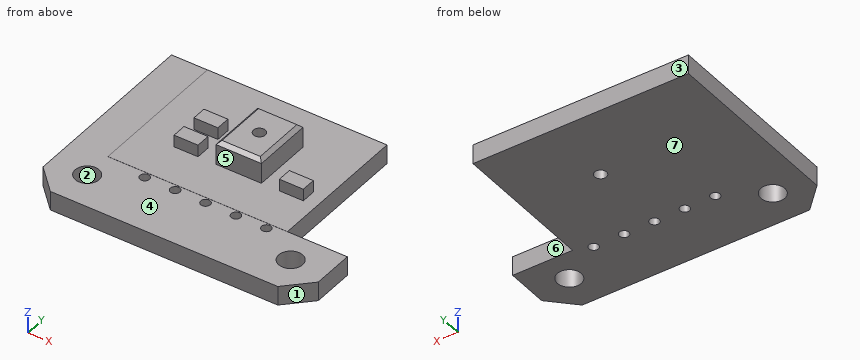
from build123d import *

# Parameters (mm, degrees)
BOSS_EXTRUDE1_DEPTH = 1.6
SKETCH2_W           = 17
SKETCH2_H           = 12
BOSS_EXTRUDE2_DEPTH = 1.61
SKETCH3_R           = 0.4
CUT_EXTRUDE1_DEPTH  = 2.62
BOSS_EXTRUDE4_START = 1.61
SKETCH4_W           = 3.8
SKETCH4_H           = 5
BOSS_EXTRUDE4_DEPTH = 2
BOSS_EXTRUDE5_START = 1.61
SKETCH5_W           = 2
SKETCH5_H           = 1.2
BOSS_EXTRUDE5_DEPTH = 1
CHAMFER1_SIZE       = 0.3
SKETCH8_R           = 1
CUT_EXTRUDE2_DEPTH  = 3.5
SKETCH9_W           = 23
SKETCH9_H           = 5.5
CUT_EXTRUDE3_DEPTH  = 3.5
SKETCH10_W          = 5
SKETCH10_H          = 12
CUT_EXTRUDE4_DEPTH  = 3.5
CUT_EXTRUDE5_START  = 3.61
SKETCH11_R          = 0.5
CUT_EXTRUDE5_DEPTH  = 5


with BuildPart() as part:
    # Sketch1 → Boss-Extrude1 (new body)
    with BuildSketch(Plane.XY):
        Polygon((-11.5, 9.5), (-9.5, 11.5), (9.5, 11.5), (11.5, 9.5), (11.5, -9.5), (9.5, -11.5), (-9.5, -11.5), (-11.5, -9.5), align=None)
    extrude(amount=BOSS_EXTRUDE1_DEPTH)

    # Sketch2 → Boss-Extrude2 (add)
    with BuildSketch(Plane.XY):
        Rectangle(SKETCH2_W, SKETCH2_H)
    extrude(amount=BOSS_EXTRUDE2_DEPTH)

    # Sketch3 → Cut-Extrude1 (cut)
    with BuildSketch(Plane.XY):
        with Locations((-5.08, -6.5)):
            Circle(SKETCH3_R)
        with Locations((-2.54, -6.5)):
            Circle(SKETCH3_R)
        with Locations((0, -6.5)):
            Circle(SKETCH3_R)
        with Locations((2.54, -6.5)):
            Circle(SKETCH3_R)
        with Locations((5.08, -6.5)):
            Circle(SKETCH3_R)
    extrude(amount=CUT_EXTRUDE1_DEPTH, mode=Mode.SUBTRACT)

    # Sketch4 → Boss-Extrude4 (add)
    with BuildSketch(Plane.XY.offset(BOSS_EXTRUDE4_START)):
        Rectangle(SKETCH4_W, SKETCH4_H)
    extrude(amount=BOSS_EXTRUDE4_DEPTH)

    # Sketch5 → Boss-Extrude5 (add)
    with BuildSketch(Plane.XY.offset(BOSS_EXTRUDE5_START)):
        with Locations((-4.4, -1.9)):
            Rectangle(SKETCH5_W, SKETCH5_H)
        with Locations((-4.4, 0.5)):
            Rectangle(SKETCH5_W, SKETCH5_H)
        with Locations((4.4, -1.9)):
            Rectangle(SKETCH5_W, SKETCH5_H)
    extrude(amount=BOSS_EXTRUDE5_DEPTH)

    # Chamfer1
    chamfer1_edges = [part.edges().sort_by_distance(p)[0] for p in [
        (1.9, 0, 3.61),
        (0, 2.5, 3.61),
        (-1.9, 0, 3.61),
        (0, -2.5, 3.61),
    ]]
    chamfer(chamfer1_edges, length=CHAMFER1_SIZE)

    # Sketch8 → Cut-Extrude2 (cut, symmetric)
    with BuildSketch(Plane.XY):
        with Locations((8.5, -8.5)):
            Circle(SKETCH8_R)
        with Locations((-8.5, -8.5)):
            Circle(SKETCH8_R)
        with Locations((8.5, 8.5)):
            Circle(SKETCH8_R)
        with Locations((-8.5, 8.5)):
            Circle(SKETCH8_R)
    extrude(amount=CUT_EXTRUDE2_DEPTH, both=True, mode=Mode.SUBTRACT)

    # Sketch9 → Cut-Extrude3 (cut, symmetric)
    with BuildSketch(Plane.XY):
        with Locations((0, 8.75)):
            Rectangle(SKETCH9_W, SKETCH9_H)
    extrude(amount=CUT_EXTRUDE3_DEPTH, both=True, mode=Mode.SUBTRACT)

    # Sketch10 → Cut-Extrude4 (cut, symmetric)
    with BuildSketch(Plane.XY):
        with Locations((9, 0)):
            Rectangle(SKETCH10_W, SKETCH10_H)
    extrude(amount=CUT_EXTRUDE4_DEPTH, both=True, mode=Mode.SUBTRACT)

    # Sketch11 → Cut-Extrude5 (cut)
    with BuildSketch(Plane.XY.offset(CUT_EXTRUDE5_START)):
        Circle(SKETCH11_R)
    extrude(amount=-CUT_EXTRUDE5_DEPTH, mode=Mode.SUBTRACT)


solid = part.part
The listing builds one solid part. Answer for the finished solid, in the listing's coordinates (mm). Face numbers are marked on the shaded views. A direction names the side the tool comes from. Coordinates: 2 decimals unless noted, no trailing zeros. Order: outer loops, then holes, each group sorted by start corner. A loop starts at its lowest first (then second) coordinate and runs counter-clockwise, first axis right, second up. Notation, with made-up numbers: (37.5, 59) -> (48.5, 59) arc R8 cw to (48.5, 74) -> close; hole circle Ø5 at (-13.5, 31). An arc over 180 degrees is marked (long way). Answer in a Markdown table with one row per item. Add a question column.
Item 1: Find section D-D (x = 0). State how many separate pieces and enclosed holes the cut face has, then the cut area to 3 significant figures.
Item 2: Each of these flat-tipped pins is pushed along its axis until it touches: P1, Ø1.8, axis at y = -2.5, z = 1, coming from the +X side; P2, Ø0.9, axis at x = 0, z = 2.5, coming from the +Y side; P3, Ø0.5, axis at x = 1, z = 2.5, coming from the -Y side; P4, Ø1.5, axis at x = -8.5, z = 2.5, coming from the -Y side. Where does it stop, or does it pass through?
Item 3: Find section B-B (z = 2.1). Write down the section's boundary in (x, y), then the cut area to 3 significant figures.
Item 4: Determine the mould class of the marked faces 1, 2 and 3 for opening direction Y: +Y half, -Y half, draft (parallel to the pull), parting line (faces both ways), or undercut.
Item 5: Find the intervals of material crossed by L1, parallel to X at y = -6.5, z = 0.7; L2, parallel to X at y = -8.5, z = 1.3; L3, parallel to Y at x = -5.08, z = 0.45, in increasing order. Write a range as from..to.
Item 6: Find section C-C (y = -6.5). Write down the section's boundary in (x, z), then the cut area to 3 significant figures.
Item 7: Which of the six approach directions +Z, -Z, +X, -X, +Y, -Y give full straight-line access (tool end or side, diameter ignored) to the marked faces 4, 5, 6 and 7?
Result set:
| question | item | result |
|---|---|---|
| 1 | separate pieces | 3 |
| 1 | enclosed holes | 0 |
| 1 | area | 33.1 mm² |
| 2 | P1 | stops at x = 6.5 |
| 2 | P2 | stops at y = 2.5 |
| 2 | P3 | stops at y = -2.5 |
| 2 | P4 | passes through |
| 3 | outline | (-5.4, -2.5) -> (-3.4, -2.5) -> (-3.4, -1.3) -> (-5.4, -1.3) -> close; (-5.4, -0.1) -> (-3.4, -0.1) -> (-3.4, 1.1) -> (-5.4, 1.1) -> close; (-1.9, -2.5) -> (1.9, -2.5) -> (1.9, 2.5) -> (-1.9, 2.5) -> close; (3.4, -2.5) -> (5.4, -2.5) -> (5.4, -1.3) -> (3.4, -1.3) -> close; hole circle Ø1 at (0, 0) |
| 3 | area | 25.4 mm² |
| 4 | face 1 | -Y half |
| 4 | face 2 | undercut |
| 4 | face 3 | +Y half |
| 5 | L1 | x = -11.5..-5.48, -4.68..-2.94, -2.14..-0.4, 0.4..2.14, 2.94..4.68, 5.48..11.5 |
| 5 | L2 | x = -11.5..-9.5, -7.5..7.5, 9.5..11.5 |
| 5 | L3 | y = -11.5..-6.9, -6.1..6 |
| 6 | outline | (-11.5, 0) -> (-5.48, 0) -> (-5.48, 1.6) -> (-11.5, 1.6) -> close; (-4.68, 0) -> (-2.94, 0) -> (-2.94, 1.6) -> (-4.68, 1.6) -> close; (-2.14, 0) -> (-0.4, 0) -> (-0.4, 1.6) -> (-2.14, 1.6) -> close; (0.4, 0) -> (2.14, 0) -> (2.14, 1.6) -> (0.4, 1.6) -> close; (2.94, 0) -> (4.68, 0) -> (4.68, 1.6) -> (2.94, 1.6) -> close; (5.48, 0) -> (11.5, 0) -> (11.5, 1.6) -> (5.48, 1.6) -> close |
| 6 | area | 30.4 mm² |
| 7 | face 4 | +Z, -X, -Y |
| 7 | face 5 | +Z, +X, -X, -Y |
| 7 | face 6 | +Z, -Z, +X, +Y |
| 7 | face 7 | -Z, +X, -X, +Y, -Y |
